from build123d import *

# Parameters (mm, degrees)
F0_W     = 300
F0_H     = 140
F1_DEPTH = 4
F2_R     = 5
F3_R     = 1
F3_R_2   = 3.5
F3_R_3   = 1.75
F3_W     = 4
F3_H     = 15
F3_R_4   = 0.75
F4_DEPTH = 4.001
F5_R     = 1
F6_DEPTH = 4.001


with BuildPart() as f1:
    # F0 (on Front) → F1 (new body)
    with BuildSketch(Plane.XZ):
        Rectangle(F0_W, F0_H)
    extrude(amount=F1_DEPTH)

    # F2
    f2_edges = [f1.edges().sort_by_distance(p)[0] for p in [
        (150, -2, 70),
        (150, -2, -70),
        (-150, -2, -70),
        (-150, -2, 70),
    ]]
    fillet(f2_edges, radius=F2_R)

    # F3 (on face) → F4 (cut, through all)
    with BuildSketch(Plane.XZ.offset(4)):
        Circle(F3_R)
        with Locations((60, 0)):
            Circle(F3_R)
        with Locations((-60, 0)):
            Circle(F3_R)
        with Locations((-110, 0)):
            Circle(F3_R_2)
        with Locations((110, 0)):
            Circle(F3_R)
        with Locations((-110, 8.5)):
            Circle(F3_R_3)
        with Locations((-110, -8.5)):
            Circle(F3_R_3)
        with Locations((-139.5, -62.5)):
            Rectangle(F3_W, F3_H)
        with Locations((139.5, -62.5)):
            Rectangle(F3_W, F3_H)
        with Locations((-145, 62)):
            Circle(F3_R_4)
        with Locations((-98.5, 62)):
            Circle(F3_R_4)
        with Locations((-145, 38.7)):
            Circle(F3_R_4)
        with Locations((-98.5, 38.7)):
            Circle(F3_R_4)
        with Locations((-20, -20)):
            Circle(F3_R)
        with Locations((20, -20)):
            Circle(F3_R)
        with Locations((20, -60)):
            Circle(F3_R)
        with Locations((-20, -60)):
            Circle(F3_R)
    extrude(amount=-F4_DEPTH, mode=Mode.SUBTRACT)

    # F5 (on face) → F6 (cut, through all)
    with BuildSketch(Plane.XZ.offset(4)):
        with Locations((0, 10)):
            Circle(F5_R)
        with Locations((0, -10)):
            Circle(F5_R)
    extrude(amount=-F6_DEPTH, mode=Mode.SUBTRACT)


solid = f1.part
Here's how the part is built. I have some questions about the finished solid (model axes, mm). Round coordinates to 2 decimals unless told otherwise and drop trailing zeros.
1. I need wall thicknesses on L1, parallel to X at y = -3.8, z = -57.5; L2, parallel to Z at x = -145, y = -1.5; L3, parallel to X at y = -2.75, z = 38.7. Which ranges of each line are inside material? Lowest first, please.
2. If we mould it in two halves opening along X, with no side actions, what happens to faces 1 (the cylindrical face through (-149, -2, -68)), 2 (the cylindrical face through (-106.767, -2.028, -1.341)), 3 (the flat face through (-2, -4, 1))? For each: released by +X, released by -X, zero draft, split by the parting line, or undercut.
3. Will these pins go through, and if not, where does the flat tip stop? pin 1 Ø2.5 at (x, z) = (-98.5, 38.7) entering from -Y; pin 2 Ø1.2 at (x, z) = (110, 0) entering from -Y.
Answer sheet:
1. L1: x = -150 to -141.5, -137.5 to 137.5, 141.5 to 150
1. L2: z = -70 to 37.95, 39.45 to 61.25, 62.75 to 70
1. L3: x = -150 to -145.75, -144.25 to -99.25, -97.75 to 150
2. face 1: released by -X
2. face 2: undercut
2. face 3: zero draft
3. pin 1: stops at y = -4
3. pin 2: passes through
